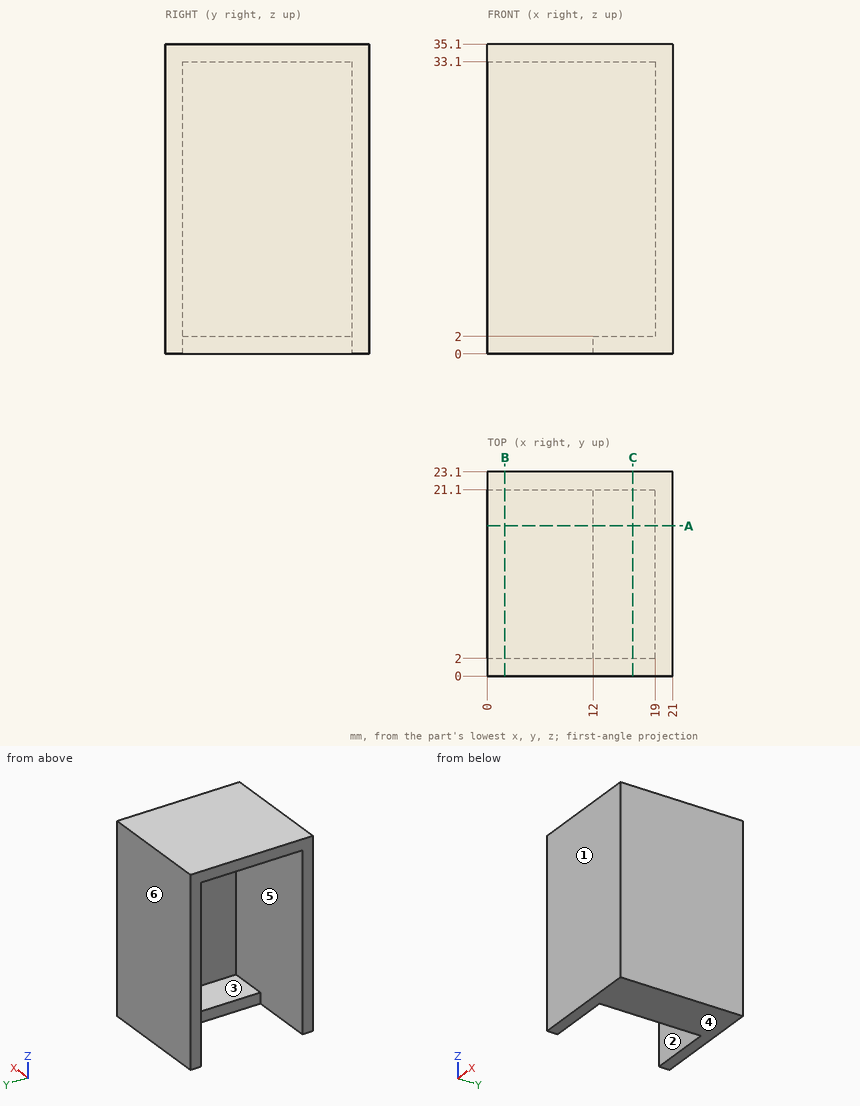
Could you check a few things on this drawing? It's one solid part, dimensions in mm from its lowest x, y, z. A direction names the side the tool comes from. Coordinates: 2 decimals unless noted, no trailing zeros. Write each loop counter-clockwise with the first axis right and the second up, starting at its lowest first coordinate (ties: lowest second). Pieces come first, ordered by that corner, then holes. Notation, with made-up numbers: (46.5, 69) - (51.5, 69) arc R12 cw to (51.5, 81) - close; hole circle Ø6 at (78.25, 56.5). An arc over 180 degrees is marked (long way). Put each result on its own line as item: value. Start each with the question number.
Q1. Which directions (+Z, -Z, +X, -X, +Y, -Y) give clear straight access to the entire face, cutting with the end or side of a thin tool? Please do the marked faces 5 and 6.
Q2. I want a section at B-B on x = 2. Write out the boundary of the cut face in (y, z), plus the area to 3 significant figures.
Q3. I want a section at C-C on x = 16.5. Write out the boundary of the cut face in (y, z).
Q4. I want a section at A-A on y = 17. Write out the boundary of the cut face in (x, z), plus the area to 3 significant figures.
Q5. Thinking about a two-plate mould opening in Y: for the marked faces 1, 2, 3 and 4, which applies, pulls with the +Y half, pulls with the -Y half, needs draft (parallel to the pull), parting line crosses it, or undercut?
Q6. I'm going to push flat-ended pins straight in: P1, Ø10, axis at x = 6, y = 11.5, coming from the -Z side; P2, Ø2, axis at y = 7.5, z = 1.5, coming from the -X side; P3, Ø3, axis at y = 16, z = 16.5, coming from the -X side. Where does each tip first touch, or does it pass through?
Q7. Please list where these lines run through material, in increasing order: L1, parallel to Z at x = 13, y = 16; L2, parallel to Y at x = 15.25, z = 19.5; L3, parallel to X at y = 4, z = 24.
Checks:
1. face 5: -X
1. face 6: +Z, -Z, +X, -X, +Y
2. outline: (0, 0) - (2, 0) - (2, 33.1) - (21.1, 33.1) - (21.1, 0) - (23.1, 0) - (23.1, 35.1) - (0, 35.1) - close
2. area: 179 mm²
3. outline: (0, 0) - (23.1, 0) - (23.1, 35.1) - (0, 35.1) - close; hole (2, 2) - (21.1, 2) - (21.1, 33.1) - (2, 33.1) - close
4. outline: (0, 33.1) - (19, 33.1) - (19, 2) - (12, 2) - (12, 0) - (21, 0) - (21, 35.1) - (0, 35.1) - close
4. area: 122 mm²
5. face 1: pulls with the -Y half
5. face 2: undercut
5. face 3: undercut
5. face 4: needs draft
6. P1: z = 33.1
6. P2: x = 12
6. P3: x = 19
7. L1: 0 to 2, 33.1 to 35.1
7. L2: 0 to 2, 21.1 to 23.1
7. L3: 19 to 21
